Source: CAD feature listing. Evaluate the final solid. Frame: model axes, mm. A direction names the side the tool comes from. Round coordinates to 2 decimals unless told otherwise and drop trailing zeros. Order: outer loops, then holes, each group sorted by start corner. A loop starts at its lowest first (then second) coordinate and runs counter-clockwise, first axis right, second up. Notation, with made-up numbers: M 22.25,85 L 34.25,85 A35 cw 34.25,121 Z; hole C -7,13 d1. An arc over 180 degrees is marked long. Answer as CSV lines item,"result". Start each with the question number.
Item 1: First-contact query: P1, Ø0.6, axis at y = -122.5, z = 5.5, coming from the +X side; P2, Ø5, axis at x = -18, z = 3, coming from the -Y side; P3, Ø4, axis at x = 26, y = -147, coming from the +Z side. Flat tips, straight axial feed; report the tip coordinate or a pass-through.
Item 2: Set-up query: faces 1 (the face through (-30, -127, 5.842)), 2 (the face through (-43.34, -161, 2)), 3 (the face through (51.91, -128, 1)), 4 (the face through (2, -133, 0)), 5 (the face through (45.56, -160, 2)). Return all of +Z, -Z, +X, -X, +Y, -Y with unobstructed straight access to the full face (end or side cutting, diameter ignored); none if empty.
Item 3: Line query: line 1 (X direction, y = -125.5, z = 5.75); line 2 (Z direction, x = 8.5, y = -132); line 3 (X direction, y = -159, z = 0.5). Output: solid intervals per line, ascending. Write a range as [from, to].
Item 4: Section query A-A on y = -118.5. Return the cut outline in (x, z), plus the area to 3 significant figures.
Item 5: Section query B-B on x = 1. Return the cut outline in (y, z), plus the area to 3 significant figures.
Item 6: Section query C-C on y = -109.5. Return the cut outline in (x, z), plus the area to 3 significant figures.
Item 7: Pull-direction query (Z, two-part tool) for faces 6 (the face through (-46, -154.045, 3)), 7 (the face through (1.732, -168.246, -1.197)), 8 (the face through (13, -132, 5.08)); classes: +Z half, -Z half, draft (parallel to the pull), parting line (faces both ways), or undercut.
Item 8: Section query D-D on x = 25. Return the cut outline in (y, z), plus the area to 3 significant figures.
from build123d import *

# Parameters (mm, degrees)
EXTRUDE1_DEPTH = 5.08
FILLET1_R      = 2.54
CHAMFER1_SIZE2 = 5.08
CHAMFER1_SIZE  = 8.798818102
EXTRUDE3_DEPTH = 88.9
SKETCH2_R      = 1.003990475
EXTRUDE2_DEPTH = 196.607873206
EXTRUDE4_DEPTH = 0.762


with BuildPart() as part:
    # Sketch1 → Extrude1 (new body)
    with BuildSketch(Plane.XY):
        Polygon((-49.690313901, -102.787097767), (51.909686099, -102.787097767), (51.909686099, -154.045409896), (45.559686099, -154.045409896), (45.559686099, -170.008151162), (-43.340313901, -170.008151162), (-43.340313901, -154.045409896), (-49.690313901, -154.045409896), align=None)
    extrude(amount=EXTRUDE1_DEPTH)

    # Fillet1
    fillet1_edges = [part.edges().sort_by_distance(p)[0] for p in [
        (51.909686099, -128.416253832, 5.08),
        (-49.690313901, -128.416253832, 5.08),
    ]]
    fillet(fillet1_edges, radius=FILLET1_R)

    # Chamfer1
    chamfer1_edges = [part.edges().sort_by_distance(p)[0] for p in [
        (1.109686099, -170.008151162, 5.08),
    ]]
    chamfer1_side = [part.faces().sort_by_distance(p)[0] for p in [
        (1.109686099, -169.906551162, 5.08),
    ]]
    chamfer(chamfer1_edges, length=CHAMFER1_SIZE - 0.0001, length2=CHAMFER1_SIZE2 - 0.0001, reference=chamfer1_side[0])  # a hair under: the kernel refuses the full size

    # Sketch3 → Extrude3 (add)
    with BuildSketch(Plane(origin=(45.559686099, 0, 0), x_dir=(0, 0, -1), z_dir=(1, 0, 0))):
        with BuildLine():
            Line((-2.656143456, -165.407575745), (0, -170.008151162))
            ThreePointArc((0, -170.008151162), (2.094834297, -170.56946032), (2.656143456, -168.474626023))
            Line((2.656143456, -168.474626023), (0, -163.874050605))
            Line((0, -163.874050605), (-2.656143456, -165.407575745))
        make_face()
    extrude(amount=-EXTRUDE3_DEPTH)

    # Sketch2 → Extrude2 (cut, through all)
    with BuildSketch(Plane(origin=(45.559686099, 0, 0), x_dir=(0, 0, -1), z_dir=(1, 0, 0))):
        with Locations((1.328071728, -169.241388592)):
            Circle(SKETCH2_R)
    extrude(amount=-EXTRUDE2_DEPTH, mode=Mode.SUBTRACT)

    # Sketch4 → Extrude4 (add)
    with BuildSketch(Plane.XY.offset(5.08)):
        with BuildLine():
            Line((2.697186099, -113.368491021), (2.697186099, -140.858908158))
            ThreePointArc((2.697186099, -140.858908158), (1.109686099, -142.446408158), (-0.477813901, -140.858908158))
            Line((-0.477813901, -140.858908158), (-0.477813901, -113.368491021))
            ThreePointArc((-0.477813901, -113.368491021), (1.109686099, -111.780991021), (2.697186099, -113.368491021))
        make_face()
        with BuildLine():
            Line((-31.531803629, -113.368491021), (-31.531803629, -140.858908158))
            ThreePointArc((-31.531803629, -140.858908158), (-29.944303629, -142.446408158), (-28.356803629, -140.858908158))
            Line((-28.356803629, -140.858908158), (-28.356803629, -113.368491021))
            ThreePointArc((-28.356803629, -113.368491021), (-29.944303629, -111.780991021), (-31.531803629, -113.368491021))
        make_face()
        with BuildLine():
            Line((33.751175827, -113.368491021), (33.751175827, -140.858908158))
            ThreePointArc((33.751175827, -140.858908158), (32.163675827, -142.446408158), (30.576175827, -140.858908158))
            Line((30.576175827, -140.858908158), (30.576175827, -113.368491021))
            ThreePointArc((30.576175827, -113.368491021), (32.163675827, -111.780991021), (33.751175827, -113.368491021))
        make_face()
    extrude(amount=EXTRUDE4_DEPTH)


solid = part.part
Results:
1,P1,"x = 33.75"
1,P2,"y = -169.14"
1,P3,"z = 5.08"
2,face 1,"+Z, +X, -X, +Y, -Y"
2,face 2,"+Z, -Z, -X, -Y"
2,face 3,"+Z, -Z, +X, +Y, -Y"
2,face 4,"-Z, +X, -X, +Y"
2,face 5,"+Z, -Z, +X, -Y"
3,line 1,"[-31.53, -28.36], [-0.48, 2.7], [30.58, 33.75]"
3,line 2,"[0, 5.08]"
3,line 3,"[-43.34, 45.56]"
4,outline,"M -49.69,0 L 51.91,0 L 51.91,2.54 A2.54 ccw 49.37,5.08 L 33.75,5.08 L 33.75,5.84 L 30.58,5.84 L 30.58,5.08 L 2.7,5.08 L 2.7,5.84 L -0.48,5.84 L -0.48,5.08 L -28.36,5.08 L -28.36,5.84 L -31.53,5.84 L -31.53,5.08 L -47.15,5.08 A2.54 ccw -49.69,2.54 Z"
4,area,"521 mm^2"
5,outline,"M -170.01,0 A1.53 ccw -168.47,-2.66 L -163.87,0 L -102.79,0 L -102.79,5.08 L -111.78,5.08 L -111.78,5.84 L -142.44,5.84 L -142.44,5.08 L -161.21,5.08 Z; hole C -169.24,-1.33 d2.01"
5,area,"351 mm^2"
6,outline,"M -49.69,0 L 51.91,0 L 51.91,2.54 A2.54 ccw 49.37,5.08 L -47.15,5.08 A2.54 ccw -49.69,2.54 Z"
6,area,"513 mm^2"
7,face 6,"draft"
7,face 7,"undercut"
7,face 8,"+Z half"
8,outline,"M -170.01,0 A1.53 ccw -168.47,-2.66 L -163.87,0 L -102.79,0 L -102.79,5.08 L -161.21,5.08 Z; hole C -169.24,-1.33 d2.01"
8,area,"328 mm^2"
